Read the model definition and answer for the solid it produces. Units are mm, in the model's axes. A direction names the side the tool comes from. Coordinates: 2 decimals unless noted, no trailing zeros. Loops run counter-clockwise (first coordinate to the right, second up) from the corner with the lowest first, then second, coordinate; pieces in that order, holes last. Notation, with made-up numbers: (70, 27.25) - (81, 27.25) arc R27 cw to (81, 58.25) - close; hole circle Ø8 at (42.25, 6.5). An arc over 180 degrees is marked (long way). Use one line per item in the form item = value.
from build123d import *

# Parameters (mm, degrees)
BOSS_EXTRUDE1_DEPTH = 3
SKETCH2_R           = 25
SKETCH2_R_2         = 17.5
BOSS_EXTRUDE2_DEPTH = 10


with BuildPart() as part:
    # Sketch1 → Boss-Extrude1 (new body)
    with BuildSketch(Plane(origin=(0, 0, 0), x_dir=(1, 0, 0), z_dir=(0, 1, 0))):
        Polygon((7.5, -62.5), (7.5, -66.5), (22.5, -66.5), (22.5, -62.5), (32.5, -62.5), (32.5, -66.5), (47.5, -66.5), (47.5, -62.5), (57.5, -62.5), (62.5, -62.5), (62.5, -59), (62.5, -47.5), (66.5, -47.5), (66.5, -32.5), (62.5, -32.5), (62.5, -22.5), (66.5, -22.5), (66.5, -7.5), (62.5, -7.5), (62.5, 7.5), (66.5, 7.5), (66.5, 22.5), (62.5, 22.5), (62.5, 32.5), (66.5, 32.5), (66.5, 47.5), (62.5, 47.5), (62.5, 59), (62.5, 62.5), (57.5, 62.5), (47.5, 62.5), (47.5, 66.5), (32.5, 66.5), (32.5, 62.5), (22.5, 62.5), (22.5, 66.5), (7.5, 66.5), (7.5, 62.5), (-7.5, 62.5), (-7.5, 66.5), (-22.5, 66.5), (-22.5, 62.5), (-32.5, 62.5), (-32.5, 66.5), (-47.5, 66.5), (-47.5, 62.5), (-59, 62.5), (-62.5, 62.5), (-62.5, 59), (-62.5, 47.5), (-66.5, 47.5), (-66.5, 32.5), (-62.5, 32.5), (-62.5, 22.5), (-66.5, 22.5), (-66.5, 7.5), (-62.5, 7.5), (-62.5, -7.5), (-66.5, -7.5), (-66.5, -22.5), (-62.5, -22.5), (-62.5, -32.5), (-66.5, -32.5), (-66.5, -47.5), (-62.5, -47.5), (-62.5, -59), (-62.5, -62.5), (-59, -62.5), (-47.5, -62.5), (-47.5, -66.5), (-32.5, -66.5), (-32.5, -62.5), (-22.5, -62.5), (-22.5, -66.5), (-7.5, -66.5), (-7.5, -62.5), align=None)
    extrude(amount=BOSS_EXTRUDE1_DEPTH)

    # Sketch2 → Boss-Extrude2 (add)
    with BuildSketch(Plane.XZ):
        Circle(SKETCH2_R)
        Circle(SKETCH2_R_2, mode=Mode.SUBTRACT)
    extrude(amount=BOSS_EXTRUDE2_DEPTH)


solid = part.part
Item 1: The part is cut by section A-A on z = 0. Give the vertices of the cut face in (x, y), plus the area to 3 significant figures.
Results below:
outline = (-62.5, 0) - (-25, 0) - (-25, -10) - (-17.5, -10) - (-17.5, 0) - (17.5, 0) - (17.5, -10) - (25, -10) - (25, 0) - (62.5, 0) - (62.5, 3) - (-62.5, 3) - close
area = 525 mm²
Item 2: Which of the six approach directions +Z, -Z, +X, -X, +Y, -Y give full straight-line access (tool end or side, diameter ignored) to faces 1 (the flat face through (64, 1, 22.5)), 2 (the flat face through (7.5, 1, 64)), 3 (the flat face through (0, 0, 0))?
Results below:
face_1 = +X, +Y, -Y
face_2 = +Z, +Y, -Y
face_3 = -Y
Item 3: The part is cut by section C-C on y = -2.5. Give the vertices of the cut face in (x, z).
Results below:
outline = circle Ø50 at (0, 0); hole circle Ø35 at (0, 0)
Item 4: Each of these flat-tipped pins is pushed along its axis until it touches: P1, Ø2.5, axis at x = -64, y = 1, coming from the +Z side; P2, Ø1.5, axis at x = 0.5, y = 1, coming from the +Z side; P3, Ø3.5, axis at y = 2, z = 65.5, coming from the +X side. Where does it stop, or does it pass through?
Results below:
P1 = 47.5
P2 = 62.5
P3 = 47.5
Item 5: The part is cut by section B-B on x = 0. Give the vertices of the cut face in (y, z).
Results below:
outline = (-10, -25) - (0, -25) - (0, -62.5) - (3, -62.5) - (3, 62.5) - (0, 62.5) - (0, 25) - (-10, 25) - (-10, 17.5) - (0, 17.5) - (0, -17.5) - (-10, -17.5) - close
Item 6: The part is cut by section D-D on x = -45. Give the vertices of the cut face in (y, z).
Results below:
outline = (0, -66.5) - (3, -66.5) - (3, 66.5) - (0, 66.5) - close
Item 7: For a pull along X with two mould halves and no side action, classify faces 4 (the flat face through (-7.5, 1, -64)), 5 (the flat face through (-65, 1, 47.5)), 6 (the flat face through (47.5, 1, -64)) as +X half, -X half, draft (parallel to the pull), parting line (faces both ways), or undercut.
Results below:
face_4 = undercut
face_5 = draft
face_6 = +X half
Item 8: Find the intervals of material crossed by L1, parallel to Z at x = 0, y = -5; L2, parallel to Y at x = -16, z = 41; L3, parallel to Z at x = -8, y = -0.5, in increasing order.
Results below:
L1 = -25 to -17.5, 17.5 to 25
L2 = 0 to 3
L3 = -23.69 to -15.56, 15.56 to 23.69
